Read the model definition and answer for the solid it produces. Units are mm, in the model's axes. Face numbers are marked on the shaded views. A direction names the side the tool comes from. Coordinates: 2 decimals unless noted, no trailing zeros. Loops run counter-clockwise (first coordinate to the right, second up) from the corner with the lowest first, then second, coordinate; pieces in that order, holes last. Notation, with made-up numbers: (38.25, -14) -> (79.25, -14) arc R8 cw to (79.25, -2) -> close; hole circle Ø11 at (70.5, 16). An arc over 180 degrees is marked (long way). Answer as a JSON object with one key per item and string values. Group by question number.
1) Section D-D, the plane z = -104 is taken. Give the vertices of the cut face in (x, y).
2) Consider probe 1 along X at (y, z) = (48.5, -115); probe 2 along X at (y, z) = (20, -12); probe 3 along Y at (x, z) = (-82, -7.5). Determine where each line is inside the solid, lowest interval first. Write a range as [from, to].
3) Section C-C, the plane x = -69.5 is taken. Give the vertices of the cut face in (y, z).
4) Section B-B, the plane y = 54 is taken. Give the vertices of the cut face in (x, z).
5) Determine the mould class of the marked faces 1, 2, 3 and 4 for opening direction X: released by +X, released by -X, zero draft, split by the parting line, or undercut.
6) Section A-A, the plane z = -128 is taken. Give the vertices of the cut face in (x, y), plus the area to 3 significant figures.
7) Flat-ended cylindrical pins translate along their axes: P1, Ø12, axis at y = 51, z = -91.5, coming from the -X side; P2, Ø25, axis at y = 22, z = -36, coming from the +X side; P3, Ø12, axis at y = 49.5, z = -102.5, coming from the +X side. Find the tip coordinate at first contact, or state that the pin passes through.
8) Which of the six approach directions +Z, -Z, +X, -X, +Y, -Y give full straight-line access (tool end or side, diameter ignored) to the marked faces 5, 6 and 7?
from build123d import *

# Parameters (mm, degrees)
IZIM1_R                     = 7.5
Y_KSEKLIK_EKSTR_ZYON1_DEPTH = 15
IZIM2_R                     = 17.5
Y_KSEKLIK_EKSTR_ZYON2_DEPTH = 15
FEDER1_REACH                = 174.399
IZIM4_WALL_W                = 417.508136348
IZIM4_WALL_H                = 10


with BuildPart() as part:
    # Çizim1 → Yükseklik-Ekstrüzyon1 (new body)
    with BuildSketch(Plane.XY):
        with BuildLine():
            Line((-142.056451613, 60.177419355), (-22.056451613, 60.177419355))
            Line((-22.056451613, 60.177419355), (-22.056451613, 10.177419355))
            ThreePointArc((-22.056451613, 10.177419355), (-27.914315989, -3.964716269), (-42.056451613, -9.822580645))
            Line((-42.056451613, -9.822580645), (-122.056451613, -9.822580645))
            ThreePointArc((-122.056451613, -9.822580645), (-136.198587237, -3.964716269), (-142.056451613, 10.177419355))
            Line((-142.056451613, 10.177419355), (-142.056451613, 60.177419355))
        make_face()
        with Locations((-122.056451613, 10.177419355)):
            Circle(IZIM1_R, mode=Mode.SUBTRACT)
        with Locations((-42.056451613, 10.177419355)):
            Circle(IZIM1_R, mode=Mode.SUBTRACT)
    extrude(amount=Y_KSEKLIK_EKSTR_ZYON1_DEPTH)

    # Çizim2 → Yükseklik-Ekstrüzyon2 (add)
    with BuildSketch(Plane(origin=(0, 60.177419355, 0), x_dir=(1, 0, 0), z_dir=(0, 1, 0))):
        with BuildLine():
            Line((-117.056451613, 115), (-117.056451613, 75))
            Line((-117.056451613, 75), (-142.056451613, 0))
            Line((-142.056451613, 0), (-22.056451613, 0))
            Line((-22.056451613, 0), (-47.056451613, 75))
            Line((-47.056451613, 75), (-47.056451613, 115))
            ThreePointArc((-47.056451613, 115), (-82.056451613, 150), (-117.056451613, 115))
        make_face()
        with Locations(Location((-82.056451613, 115, 0), (0, 0, 270))):
            Circle(IZIM2_R, mode=Mode.SUBTRACT)
    extrude(amount=-Y_KSEKLIK_EKSTR_ZYON2_DEPTH)

    # Çizim4 wall → Feder1 (add, up to next)
    with BuildSketch(Plane(origin=(-82.056451613, 20.177419355, -25), x_dir=(0, 0.707106781187, -0.707106781187), z_dir=(0, -0.707106781187, -0.707106781187)), mode=Mode.PRIVATE) as feder1_sk1:
        Rectangle(IZIM4_WALL_W, IZIM4_WALL_H)
    feder1_tool1 = extrude(feder1_sk1.sketch, amount=-FEDER1_REACH, mode=Mode.PRIVATE) - part.part
    add(feder1_tool1.solids().sort_by_distance((-82.056451613, 20.177419355, -25))[0])


solid = part.part
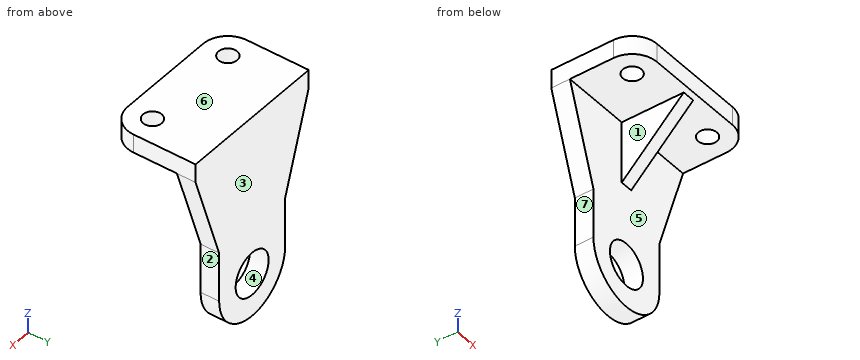
Determined:
{
 "1": {"outline": "(-117.06, 45.18) -> (-95.67, 45.18) -> (-95.67, 60.18) -> (-117.06, 60.18) -> close; (-68.45, 45.18) -> (-47.06, 45.18) -> (-47.06, 60.18) -> (-68.45, 60.18) -> close"},
 "2": {"probe 1": "[-117.06, -99.56], [-64.56, -47.06]", "probe 2": "[-87.06, -77.06]", "probe 3": "[2.68, 60.18]"},
 "3": {"outline": "(-9.82, 0) -> (45.18, 0) -> (45.18, -102.81) -> (60.18, -102.81) -> (60.18, 15) -> (-9.82, 15) -> close; (45.18, -147.67) -> (60.18, -147.67) -> (60.18, -127.19) -> (45.18, -127.19) -> close"},
 "4": {"outline": "(-142.06, 0) -> (-117.06, -75) -> (-117.06, -115) arc R35 ccw to (-47.06, -115) -> (-47.06, -75) -> (-22.06, 0) -> (-22.06, 15) -> (-142.06, 15) -> close; hole circle Ø35 at (-82.06, -115)"},
 "5": {"face 1": "released by -X", "face 2": "released by +X", "face 3": "zero draft", "face 4": "undercut"},
 "6": {"outline": "(-114.55, 45.18) -> (-93.77, 45.18) -> (-93.77, 60.18) -> (-114.55, 60.18) -> close; (-70.34, 45.18) -> (-49.56, 45.18) -> (-49.56, 60.18) -> (-70.34, 60.18) -> close", "area": "623 mm²"},
 "7": {"P1": "x = -117.06", "P2": "x = -77.06", "P3": "x = -47.06"},
 "8": {"face 5": "-Z, -Y", "face 6": "+Z, +X, -X, +Y, -Y", "face 7": "-Z, -X, +Y, -Y"}
}
